Here's how the part is built. I have some questions about the finished solid (model axes, mm). Round coordinates to 2 decimals unless told otherwise and drop trailing zeros. Loops run counter-clockwise (first coordinate to the right, second up) from the corner with the lowest first, then second, coordinate; pieces in that order, holes last. Notation, with made-up numbers: M 12,-9.75 L 63,-9.75 A25 ccw 63,18.25 Z; hole C 58,68.25 d11. An arc over 180 degrees is marked long. Answer as a JSON object with one key per item and string values.
from build123d import *

# Parameters (mm, degrees)
SKETCH1_R             = 33.8
SKETCH1_R_2           = 2.54
SKETCH1_R_3           = 2.05
SKETCH1_W             = 3.048
SKETCH1_H             = 19.05
SKETCH1_W_2           = 19.05
SKETCH1_H_2           = 3.048
BOSS_EXTRUDE1_DEPTH   = 3.175
BOSS_EXTRUDE2_DEPTH   = 3.175
FILLET1_R             = 2.54
SKETCH4_R             = 33.927
SKETCH4_R_2           = 2.413
SKETCH4_R_3           = 1.923
SKETCH4_W             = 2.794
SKETCH4_H             = 18.796
SKETCH4_W_2           = 18.796
SKETCH4_H_2           = 2.794
KERF_ADJUSTMENT_DEPTH = 3.175


with BuildPart() as part:
    # Sketch1 → Boss-Extrude1 (new body)
    with BuildSketch(Plane.XY):
        Circle(SKETCH1_R)
        with Locations((14.36, 24.872249597)):
            Circle(SKETCH1_R_2, mode=Mode.SUBTRACT)
        with Locations((20.308106756, 20.308106756)):
            Circle(SKETCH1_R_2, mode=Mode.SUBTRACT)
        with Locations((24.872249597, 14.36)):
            Circle(SKETCH1_R_2, mode=Mode.SUBTRACT)
        with Locations((27.741389731, 7.433282975)):
            Circle(SKETCH1_R_2, mode=Mode.SUBTRACT)
        with Locations((28.72, 0)):
            Circle(SKETCH1_R_2, mode=Mode.SUBTRACT)
        with Locations((27.741389731, -7.433282975)):
            Circle(SKETCH1_R_2, mode=Mode.SUBTRACT)
        with Locations((24.872249597, -14.36)):
            Circle(SKETCH1_R_2, mode=Mode.SUBTRACT)
        with Locations((20.308106756, -20.308106756)):
            Circle(SKETCH1_R_2, mode=Mode.SUBTRACT)
        with Locations((14.36, -24.872249597)):
            Circle(SKETCH1_R_2, mode=Mode.SUBTRACT)
        with Locations((7.433282975, -27.741389731)):
            Circle(SKETCH1_R_2, mode=Mode.SUBTRACT)
        with Locations((0, -28.72)):
            Circle(SKETCH1_R_2, mode=Mode.SUBTRACT)
        with Locations((-7.433282975, -27.741389731)):
            Circle(SKETCH1_R_2, mode=Mode.SUBTRACT)
        with Locations((-14.36, -24.872249597)):
            Circle(SKETCH1_R_2, mode=Mode.SUBTRACT)
        with Locations((-20.308106756, -20.308106756)):
            Circle(SKETCH1_R_2, mode=Mode.SUBTRACT)
        with Locations((-24.872249597, -14.36)):
            Circle(SKETCH1_R_2, mode=Mode.SUBTRACT)
        with Locations((-27.741389731, -7.433282975)):
            Circle(SKETCH1_R_2, mode=Mode.SUBTRACT)
        with Locations((-28.72, 0)):
            Circle(SKETCH1_R_2, mode=Mode.SUBTRACT)
        with Locations((-27.741389731, 7.433282975)):
            Circle(SKETCH1_R_2, mode=Mode.SUBTRACT)
        with Locations((-24.872249597, 14.36)):
            Circle(SKETCH1_R_2, mode=Mode.SUBTRACT)
        with Locations((-20.308106756, 20.308106756)):
            Circle(SKETCH1_R_2, mode=Mode.SUBTRACT)
        with Locations((-14.36, 24.872249597)):
            Circle(SKETCH1_R_2, mode=Mode.SUBTRACT)
        with Locations((-7.433282975, 27.741389731)):
            Circle(SKETCH1_R_2, mode=Mode.SUBTRACT)
        with Locations((0, 28.72)):
            Circle(SKETCH1_R_2, mode=Mode.SUBTRACT)
        with Locations((7.433282975, 27.741389731)):
            Circle(SKETCH1_R_2, mode=Mode.SUBTRACT)
        Circle(SKETCH1_R_3, mode=Mode.SUBTRACT)
        with Locations((0, 14.115)):
            Rectangle(SKETCH1_W, SKETCH1_H, mode=Mode.SUBTRACT)
        with Locations((14.115, 0)):
            Rectangle(SKETCH1_W_2, SKETCH1_H_2, mode=Mode.SUBTRACT)
        with Locations((0, -14.115)):
            Rectangle(SKETCH1_W, SKETCH1_H, mode=Mode.SUBTRACT)
        with Locations((-14.115, 0)):
            Rectangle(SKETCH1_W_2, SKETCH1_H_2, mode=Mode.SUBTRACT)
    extrude(amount=BOSS_EXTRUDE1_DEPTH)

    # Sketch3 → Boss-Extrude2 (add)
    with BuildSketch(Plane.XY):
        with BuildLine():
            Line((-2.694076836, 35.224076836), (-4.406640425, 33.511513248))
            ThreePointArc((-4.406640425, 33.511513248), (0, 33.8), (4.406640425, 33.511513248))
            Line((4.406640425, 33.511513248), (2.694076836, 35.224076836))
            ThreePointArc((2.694076836, 35.224076836), (0, 36.34), (-2.694076836, 35.224076836))
        make_face()
    extrude(amount=BOSS_EXTRUDE2_DEPTH)

    # Fillet1
    fillet1_edges = [part.edges().sort_by_distance(p)[0] for p in [
        (-4.406640425, 33.511513248, 1.5875),
        (4.406640425, 33.511513248, 1.5875),
    ]]
    fillet(fillet1_edges, radius=FILLET1_R)

    # Sketch4 → Kerf Adjustment (add)
    with BuildSketch(Plane.XY):
        Circle(SKETCH4_R)
        with Locations((28.72, 0)):
            Circle(SKETCH4_R_2, mode=Mode.SUBTRACT)
        with Locations((27.741389731, 7.433282975)):
            Circle(SKETCH4_R_2, mode=Mode.SUBTRACT)
        with Locations((24.872249597, 14.36)):
            Circle(SKETCH4_R_2, mode=Mode.SUBTRACT)
        with Locations((20.308106756, 20.308106756)):
            Circle(SKETCH4_R_2, mode=Mode.SUBTRACT)
        with Locations((-14.36, -24.872249597)):
            Circle(SKETCH4_R_2, mode=Mode.SUBTRACT)
        with Locations((-7.433282975, -27.741389731)):
            Circle(SKETCH4_R_2, mode=Mode.SUBTRACT)
        with Locations((0, -28.72)):
            Circle(SKETCH4_R_2, mode=Mode.SUBTRACT)
        with Locations((7.433282975, -27.741389731)):
            Circle(SKETCH4_R_2, mode=Mode.SUBTRACT)
        with Locations((14.36, -24.872249597)):
            Circle(SKETCH4_R_2, mode=Mode.SUBTRACT)
        with Locations((20.308106756, -20.308106756)):
            Circle(SKETCH4_R_2, mode=Mode.SUBTRACT)
        with Locations((24.872249597, -14.36)):
            Circle(SKETCH4_R_2, mode=Mode.SUBTRACT)
        with Locations((27.741389731, -7.433282975)):
            Circle(SKETCH4_R_2, mode=Mode.SUBTRACT)
        with Locations((-14.36, 24.872249597)):
            Circle(SKETCH4_R_2, mode=Mode.SUBTRACT)
        with Locations((-20.308106756, 20.308106756)):
            Circle(SKETCH4_R_2, mode=Mode.SUBTRACT)
        with Locations((-24.872249597, 14.36)):
            Circle(SKETCH4_R_2, mode=Mode.SUBTRACT)
        with Locations((-27.741389731, 7.433282975)):
            Circle(SKETCH4_R_2, mode=Mode.SUBTRACT)
        with Locations((-28.72, 0)):
            Circle(SKETCH4_R_2, mode=Mode.SUBTRACT)
        with Locations((-27.741389731, -7.433282975)):
            Circle(SKETCH4_R_2, mode=Mode.SUBTRACT)
        with Locations((-24.872249597, -14.36)):
            Circle(SKETCH4_R_2, mode=Mode.SUBTRACT)
        with Locations((-20.308106756, -20.308106756)):
            Circle(SKETCH4_R_2, mode=Mode.SUBTRACT)
        Circle(SKETCH4_R_3, mode=Mode.SUBTRACT)
        with Locations((7.433282975, 27.741389731)):
            Circle(SKETCH4_R_2, mode=Mode.SUBTRACT)
        with Locations((0, 28.72)):
            Circle(SKETCH4_R_2, mode=Mode.SUBTRACT)
        with Locations((-7.433282975, 27.741389731)):
            Circle(SKETCH4_R_2, mode=Mode.SUBTRACT)
        with Locations((14.36, 24.872249597)):
            Circle(SKETCH4_R_2, mode=Mode.SUBTRACT)
        with Locations((0, -14.115)):
            Rectangle(SKETCH4_W, SKETCH4_H, mode=Mode.SUBTRACT)
        with Locations((14.115, 0)):
            Rectangle(SKETCH4_W_2, SKETCH4_H_2, mode=Mode.SUBTRACT)
        with Locations((0, 14.115)):
            Rectangle(SKETCH4_W, SKETCH4_H, mode=Mode.SUBTRACT)
        with Locations((-14.115, 0)):
            Rectangle(SKETCH4_W_2, SKETCH4_H_2, mode=Mode.SUBTRACT)
    extrude(amount=KERF_ADJUSTMENT_DEPTH)


solid = part.part
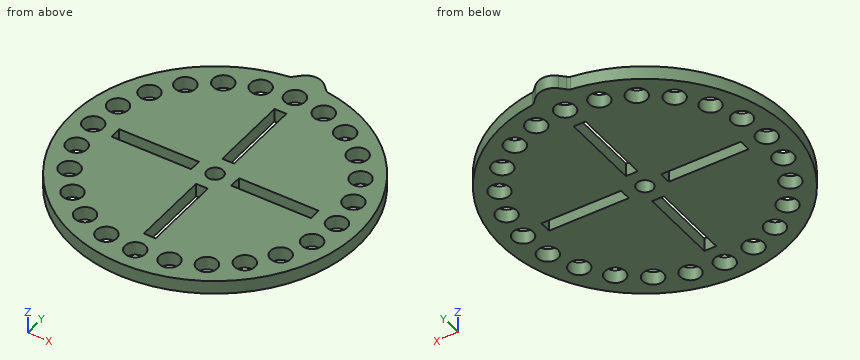
Item 1: I want a section at C-C on x = 14.36. List the corners of the cut face in (y, z) for me (3 decimals).
Solution:
{"outline": "M -30.738,0 L -27.285,0 L -27.285,3.175 L -30.738,3.175 Z; M -22.459,0 L -1.397,0 L -1.397,3.175 L -22.459,3.175 Z; M 1.397,0 L 22.459,0 L 22.459,3.175 L 1.397,3.175 Z; M 27.285,0 L 30.738,0 L 30.738,3.175 L 27.285,3.175 Z"}
Item 2: I want a section at D-D on z = 1.75. Count the separate pieces of the cut face and the enclosed holes in it, plus the area to 3 significant figures.
Solution:
{"separate pieces": "1", "enclosed holes": "29", "area": "2,970 mm2"}
Item 3: I want a section at A-A on x = 0. List the corners of the cut face in (y, z) for me (3 decimals).
Solution:
{"outline": "M -33.927,0 L -31.133,0 L -31.133,3.175 L -33.927,3.175 Z; M -26.307,0 L -23.513,0 L -23.513,3.175 L -26.307,3.175 Z; M -4.717,0 L -1.923,0 L -1.923,3.175 L -4.717,3.175 Z; M 1.923,0 L 4.717,0 L 4.717,3.175 L 1.923,3.175 Z; M 23.513,0 L 26.307,0 L 26.307,3.175 L 23.513,3.175 Z; M 31.133,0 L 36.34,0 L 36.34,3.175 L 31.133,3.175 Z"}
Item 4: For P1, Ø0.8, axis at x = -0.5, z = 1, coming from the -Y side; P2, Ø1, axis at x = 2.5, z = 1, coming from the +Y side, each with a flat end and sliding along its axis, tell me the tip position at first contact or that it passes through.
Solution:
{"P1": "stops at y = -33.93", "P2": "stops at y = 35.77"}
Item 5: If I drill on L1, parallel to Y at x = -14.36, z = 1.4; L2, parallel to Y at x = -21, z = 0.95; L3, parallel to X at y = -5.5, z = 2.25, over which ranges is the centre line in solid material (lowest first)? Write a range as from..to.
Solution:
{"L1": "y = -30.74..-27.29, -22.46..-1.4, 1.4..22.46, 27.29..30.74", "L2": "y = -26.65..-22.62, -18..-1.4, 1.4..18, 22.62..26.65", "L3": "x = -33.48..-29.19, -26.3..-1.4, 1.4..26.3, 29.19..33.48"}
Item 6: I want a section at B-B on y = 28.72. List the corners of the cut face in (x, z) for me (3 decimals), plus the area to 3 significant figures.
Solution:
{"outline": "M -18.061,0 L -9.639,0 L -9.639,3.175 L -18.061,3.175 Z; M -5.228,0 L -2.413,0 L -2.413,3.175 L -5.228,3.175 Z; M 2.413,0 L 5.228,0 L 5.228,3.175 L 2.413,3.175 Z; M 9.639,0 L 18.061,0 L 18.061,3.175 L 9.639,3.175 Z", "area": "71.4 mm2"}
